Design review of the part built by this model. Coordinates are the model's own, in mm. Face numbers are marked on the shaded views. Give positions to 0.01 mm unless a question says otherwise; leave off trailing zeros. Order: outer loops, then holes, each group sorted by start corner. A loop starts at its lowest first (then second) coordinate and runs counter-clockwise, first axis right, second up.
```python
from build123d import *

# Parameters (mm, degrees)
F0_R     = 21.5
F1_DEPTH = 12
F3_D     = 35
F5_D     = 2
F5_DEPTH = 10
F5_TIP   = 0.600860619


with BuildPart() as f1:
    # F0 (on Top) → F1 (new body)
    with BuildSketch(Plane.XY):
        Circle(F0_R)
    extrude(amount=F1_DEPTH)

    # F3 (through all)
    with Locations(Plane.XY.offset(12)):
        with Locations((0, 0)):
            Hole(F3_D / 2)

    # F5
    with Locations(Plane.XY.offset(12)):
        with Locations((-13.7885822331, 13.7885822331), (13.7885822331, 13.7885822331), (13.7885822331, -13.7885822331), (-13.7885822331, -13.7885822331)):
            Hole(F5_D / 2, depth=F5_DEPTH)
            with Locations((0, 0, -(F5_DEPTH + F5_TIP / 2))):  # 118° drill point
                Cone(0, F5_D / 2, F5_TIP, mode=Mode.SUBTRACT)


solid = f1.part
```
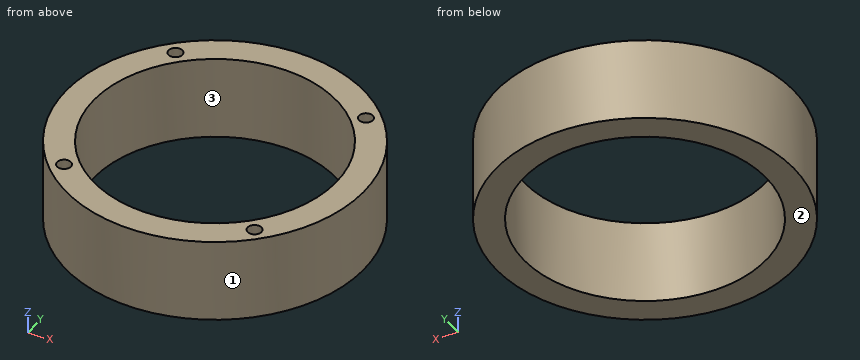
1. Take a section at C-C (z = 7.75). State the section outline as (x, y) points.
Recorded:
outline: circle Ø43 at (0, 0); hole circle Ø35 at (0, 0); hole circle Ø2 at (-13.79, -13.79); hole circle Ø2 at (-13.79, 13.79); hole circle Ø2 at (13.79, -13.79); hole circle Ø2 at (13.79, 13.79)
2. Draft analysis for pull direction X (two halves, no side actions). For the marked faces 1, 2 and 3, state which applies: pulls with the +X half, pulls with the -X half, needs draft (parallel to the pull), parting line crosses it, or undercut.
Recorded:
face 1: parting line crosses it
face 2: needs draft
face 3: undercut
3. For pin 1 (1 mm diameter, centred on x = -11.5, z = 5, fed in from +Y); pin 2 (5 mm diameter, centred on y = -5.5, z = 8, fed in from -X), all flat-tipped, find the tip position at first contact; note any pin that passes through.
Recorded:
pin 1: stops at y = 18.47
pin 2: stops at x = -21.29
4. Take a section at A-A (y = 0). State the section outline as (x, z) points, then the cut area to 3 significant figures.
Recorded:
outline: (-21.5, 0) - (-17.5, 0) - (-17.5, 12) - (-21.5, 12) - close; (17.5, 0) - (21.5, 0) - (21.5, 12) - (17.5, 12) - close
area: 96.0 mm2
5. For line 1 along X through (y, z) = (-0.5, 3.5); line 2 along Y through (x, z) = (0, 7.5); line 3 along Y through (x, z) = (8.5, 8.25), list the stretches that pass through material, from the lowest coordinate up.
Recorded:
line 1: x = -21.49 to -17.49, 17.49 to 21.49
line 2: y = -21.5 to -17.5, 17.5 to 21.5
line 3: y = -19.75 to -15.3, 15.3 to 19.75
